Can you work these out from the drawing? Everything is in mm from the part's minimum corner. Round coordinates to 2 decimals unless told otherwise and drop trailing zeros. Order: outer loops, then holes, each group sorted by start corner. A loop starts at its lowest first (then second) coordinate and runs counter-clockwise, first axis right, second up. Notation, with made-up numbers: (53, 85) -> (81, 85) arc R33 ccw to (81, 122) -> close; hole circle Ø4 at (59.5, -17). An arc over 180 degrees is marked (long way). Use a Markdown table: item, result. Add a question column.
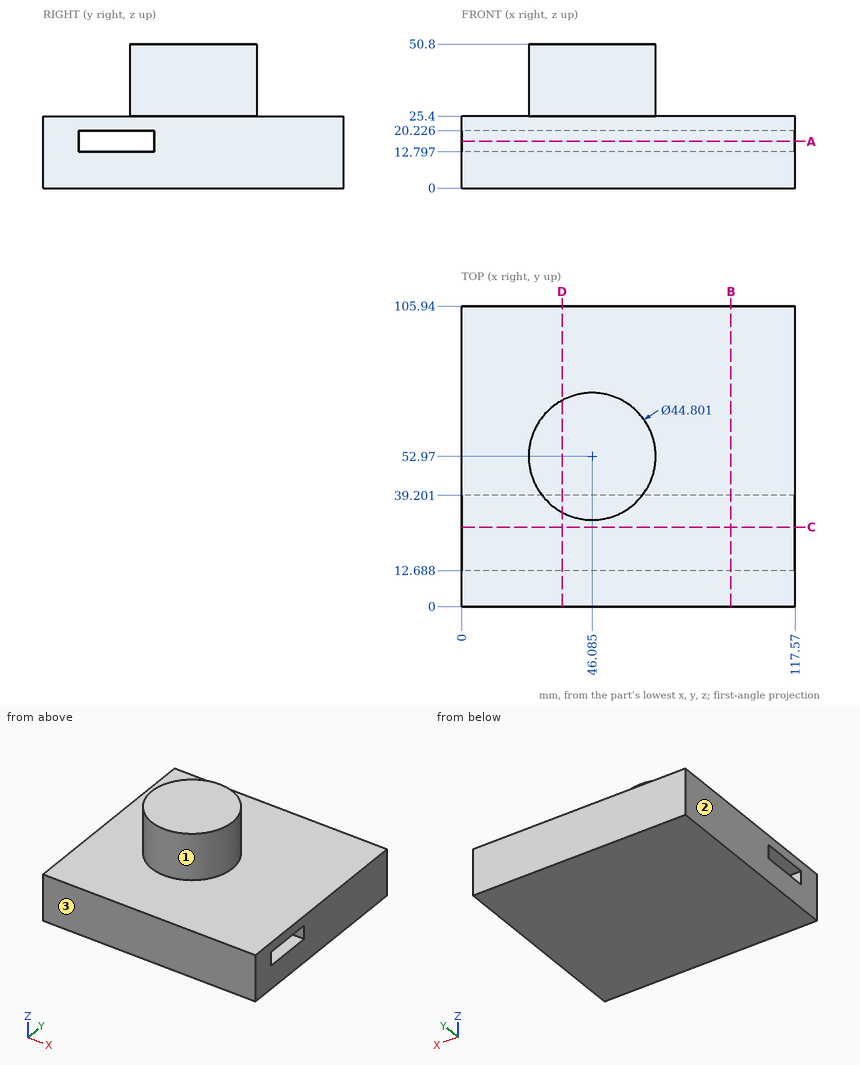
(1) I want a section at C-C on y = 28. List the corners of the cut face in (x, z) for me.
(2) I want a section at B-B on x = 95. List the corners of the cut face in (y, z) for me, and give its area (3 significant figures).
(3) I want a section at A-A on z = 16.5. List the corners of the cut face in (x, y) for me, and give its area (3 significant figures).
(4) I'm going to push a flat-ended pin straight in: P1, Ø3, axis at x = 12.5, y = 31, coming from the +Z side. Where does the tip first touch, or does it pass through?
(5) Please list where these lines run through material, in increasing order: probe 1 along Z at (x, y) = (16.5, 24.5); probe 2 along Y at (x, z) = (31, 14.5); probe 3 along Z at (x, y) = (94, 91). Write a range as from..to.
(6) I want a section at D-D on x = 35.5. List the corners of the cut face in (y, z) for me.
(7) If we mould it in two halves opening along X, with no side actions, what happens to the marked faces 1, 2 and 3? For each: pulls with the +X half, pulls with the -X half, needs draft (parallel to the pull), parting line crosses it, or undercut.
Output:
| question | item | result |
|---|---|---|
| 1 | outline | (0, 0) -> (117.57, 0) -> (117.57, 12.8) -> (0, 12.8) -> close; (0, 20.23) -> (117.57, 20.23) -> (117.57, 25.4) -> (0, 25.4) -> close |
| 2 | outline | (0, 0) -> (105.94, 0) -> (105.94, 25.4) -> (0, 25.4) -> close; hole (12.69, 12.8) -> (39.2, 12.8) -> (39.2, 20.23) -> (12.69, 20.23) -> close |
| 2 | area | 2,490 mm² |
| 3 | outline | (0, 0) -> (117.57, 0) -> (117.57, 12.69) -> (0, 12.69) -> close; (0, 39.2) -> (117.57, 39.2) -> (117.57, 105.94) -> (0, 105.94) -> close |
| 3 | area | 9,340 mm² |
| 4 | P1 | z = 25.4 |
| 5 | probe 1 | 0..12.8, 20.23..25.4 |
| 5 | probe 2 | 0..12.69, 39.2..105.94 |
| 5 | probe 3 | 0..25.4 |
| 6 | outline | (0, 0) -> (105.94, 0) -> (105.94, 25.4) -> (72.71, 25.4) -> (72.71, 50.8) -> (33.23, 50.8) -> (33.23, 25.4) -> (0, 25.4) -> close; hole (12.69, 12.8) -> (39.2, 12.8) -> (39.2, 20.23) -> (12.69, 20.23) -> close |
| 7 | face 1 | parting line crosses it |
| 7 | face 2 | pulls with the -X half |
| 7 | face 3 | needs draft |
